Geometry check sheet. Reference: drawing and pictorial views, mm from the part's lowest x, y, z. A direction names the side the tool comes from. Give positions to 0.01 mm unless a question says otherwise; leave off trailing zeros. Order: outer loops, then holes, each group sorted by start corner. A loop starts at its lowest first (then second) coordinate and runs counter-clockwise, first axis right, second up. Notation, with made-up numbers: (57.5, -5.75) -> (62.5, -5.75) arc R23 cw to (62.5, 23.25) -> close; hole circle Ø2 at (64, 9). An arc over 180 degrees is marked (long way). Write each question's results on one line, items separated by ' | '.
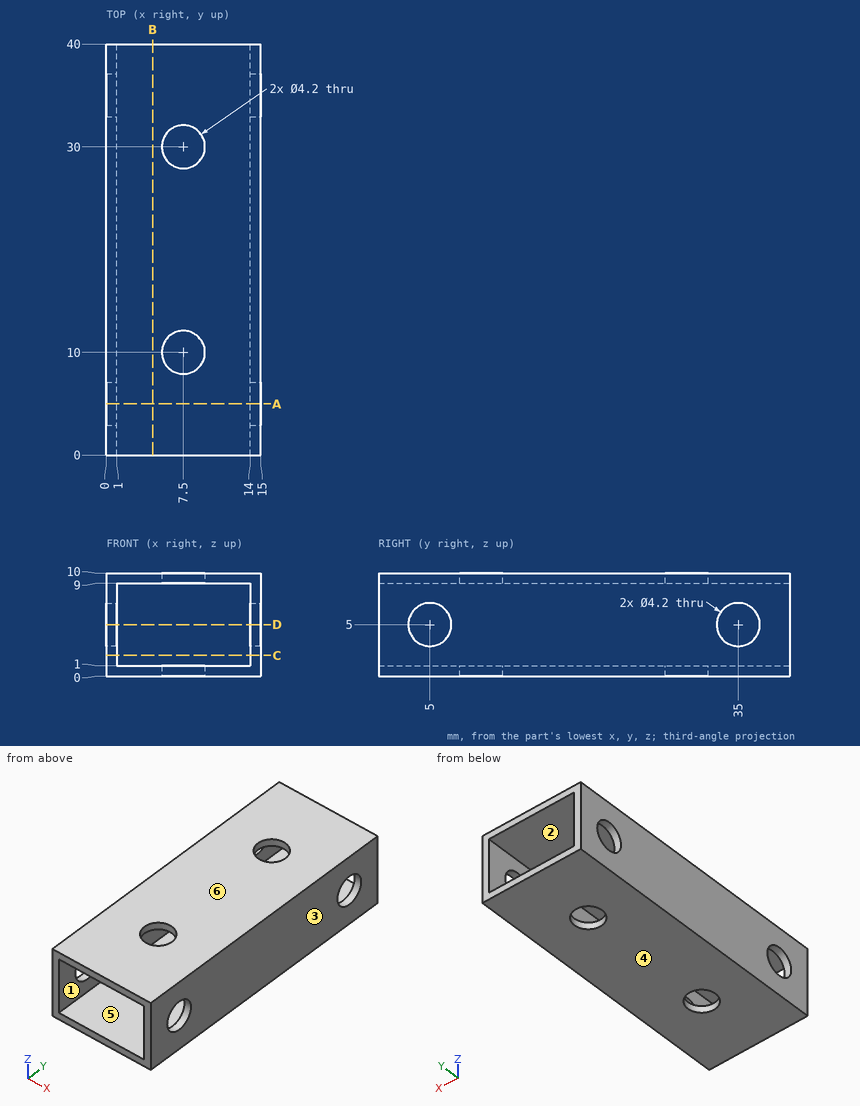
1. Mould release check, pull along Z, two halves, no side actions. Record for the marked faces 1, 2, 3 and 4: +Z half, -Z half, draft (parallel to the pull), parting line (faces both ways), or undercut.
Verdict:
face 1: undercut | face 2: undercut | face 3: draft | face 4: -Z half
2. Access from +Z, -Z, +X, -X, +Y, -Y to the whole of each face (thin tool, end or side, straight path). Record for the marked faces 5 and 6.
Verdict:
face 5: +Y, -Y | face 6: +Z, +X, -X, +Y, -Y
3. Section check B-B on x = 4.5. Record the cut outline in (y, z), then the cut area to 3 significant figures.
Verdict:
outline: (0, 0) -> (40, 0) -> (40, 1) -> (0, 1) -> close; (0, 9) -> (40, 9) -> (40, 10) -> (0, 10) -> close | area: 80.0 mm^2
4. Section check A-A on y = 5. Record the cut outline in (x, z), then the cut area to 3 significant figures.
Verdict:
outline: (0, 0) -> (15, 0) -> (15, 2.9) -> (14, 2.9) -> (14, 1) -> (1, 1) -> (1, 2.9) -> (0, 2.9) -> close; (0, 7.1) -> (1, 7.1) -> (1, 9) -> (14, 9) -> (14, 7.1) -> (15, 7.1) -> (15, 10) -> (0, 10) -> close | area: 37.6 mm^2
5. Material ranges on probe 1 along Y at (x, z) = (7.5, 9.65); probe 2 along X at (y, z) = (14.5, 8); probe 3 along Z at (x, y) = (10.25, 4.5), recorded low to high. Write a range as from..to.
Verdict:
probe 1: y = 0..7.9, 12.1..27.9, 32.1..40 | probe 2: x = 0..1, 14..15 | probe 3: z = 0..1, 9..10
6. Section check C-C on z = 2. Record the cut outline in (x, y), then the cut area to 3 significant figures.
Verdict:
outline: (0, 0) -> (1, 0) -> (1, 40) -> (0, 40) -> close; (14, 0) -> (15, 0) -> (15, 40) -> (14, 40) -> close | area: 80.0 mm^2
7. Section check D-D on z = 5. Record the cut outline in (x, y), then the cut area to 3 significant figures.
Verdict:
outline: (0, 0) -> (1, 0) -> (1, 2.9) -> (0, 2.9) -> close; (0, 7.1) -> (1, 7.1) -> (1, 32.9) -> (0, 32.9) -> close; (0, 37.1) -> (1, 37.1) -> (1, 40) -> (0, 40) -> close; (14, 0) -> (15, 0) -> (15, 2.9) -> (14, 2.9) -> close; (14, 7.1) -> (15, 7.1) -> (15, 32.9) -> (14, 32.9) -> close; (14, 37.1) -> (15, 37.1) -> (15, 40) -> (14, 40) -> close | area: 63.2 mm^2
